Autodesk Fusion 360 part; units mm, degrees
sketch "Sketch2" plane through (0, 0, 0) normal (0, 0, -1) x (1, 0, 0)
  arc A0 (124, -92) -> (125, -91) centre (124, -91) ccw
  line L0 (125, -91) -> (125, -1)
  arc A1 (125, -1) -> (124, 0) centre (124, -1) ccw
  line L1 (124, 0) -> (1, 0)
  arc A2 (1, 0) -> (0, -1) centre (1, -1) ccw
  line L2 (0, -1) -> (0, -91)
  arc A3 (0, -91) -> (1, -92) centre (1, -91) ccw
  line L3 (1, -92) -> (124, -92)
  circle A4 centre (54.1, -72.1) radius 1
  circle A5 centre (11, -21.3) radius 1
  circle A6 centre (26.2, -72.1) radius 1
  circle A7 centre (59.2, -20) radius 1
extrude "Extrude1" add sketch "Sketch2" along normal blind 6
sketch "Sketch1" plane through (0, 0, -6) normal (0, 0, -1) x (1, 0, 0)
  circle A0 centre (59.2, -20) radius 1
  circle A1 centre (11, -21.3) radius 1
  circle A2 centre (26.2, -72.1) radius 1
  circle A3 centre (54.1, -72.1) radius 1
  line L0 (1, -92) -> (124, -92)
  arc A4 (124, -92) -> (125, -91) centre (124, -91) ccw
  line L1 (125, -91) -> (125, -1)
  arc A5 (125, -1) -> (124, 0) centre (124, -1) ccw
  line L2 (124, 0) -> (1, 0)
  arc A6 (1, 0) -> (0, -1) centre (1, -1) ccw
  line L3 (0, -1) -> (0, -91)
  arc A7 (0, -91) -> (1, -92) centre (1, -91) ccw
  line L4 (0, -15) -> (125, -15)
  line L5 (125, -15) -> (125, -25)
  line L6 (125, -25) -> (0, -25)
  line L7 (0, -25) -> (0, -15)
  line L8 (0, -67) -> (125, -67)
  line L9 (125, -67) -> (125, -77)
  line L10 (125, -77) -> (0, -77)
  line L11 (0, -77) -> (0, -67)
  dimension "d215" = 15
  dimension "d216" = 10
  dimension "d217" = 15
  dimension "d218" = 10
extrude "Extrude2" cut sketch "Sketch1" against normal blind 3 contours L1 L3 L8 L9 L10 L11 | L1 L3 L4 L5 L6 L7
fillet "Fillet1" radius 3 1 edges at (125, 20, -3)
fillet "Fillet2" radius 3 1 edges at (125, 72, -3)
fillet "Fillet3" radius 3 1 edges at (0, 72, -3)
fillet "Fillet4" radius 3 1 edges at (0, 20, -3)
delete_face "DeleteFace1" 1 faces at (60.1215, 19.6116, -2)
delete_face "DeleteFace2" 1 faces at (11.995, 21.3996, -1)
delete_face "DeleteFace3" 1 faces at (25.2198, 71.9019, -2)
delete_face "DeleteFace4" 1 faces at (55.0691, 71.8532, -2)
hole "Hole1" at (62.5, 46, 0) direction (0, 0, -1) diameter 2.5 end through all countersink diameter 7.5 countersink angle 90
hole "Hole2" at (62.5, 7.5, 0) direction (0, 0, -1) diameter 2.5 end through all countersink diameter 7.5 countersink angle 90
hole "Hole3" at (62.5, 84.5, 0) direction (0, 0, -1) diameter 2.5 end through all countersink diameter 7.5 countersink angle 90
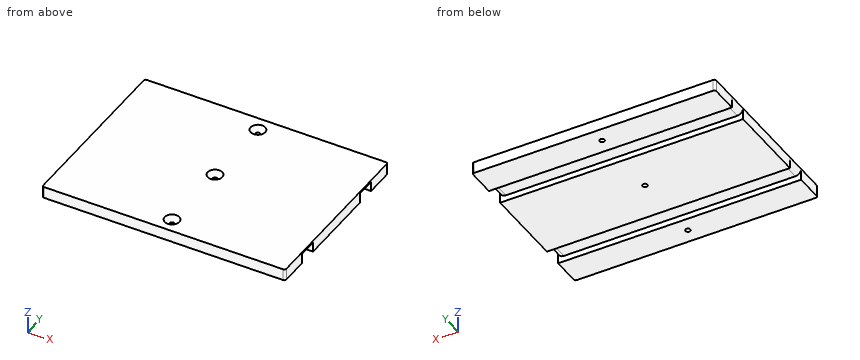
Geometry: final body of the model. Coordinates: model frame, mm. Round coordinates to 2 decimals unless told otherwise and drop trailing zeros. Order: outer loops, then holes, each group sorted by start corner. A loop starts at its lowest first (then second) coordinate and runs counter-clockwise, first axis right, second up. Notation, with made-up numbers: M -21.5,75.5 L 6.5,75.5 A14 cw 6.5,100.5 Z; hole C 5.5,-22 d10. An arc over 180 degrees is marked long. One line per item, written item: value.
(1) Cut plane B-B (y = 46). Return the cut outline in (x, z), and give its area (3 significant figures).
Result sheet:
outline: M 0,-6 L 61.25,-6 L 61.25,-2.5 L 58.75,0 L 0,0 Z; M 63.75,-6 L 125,-6 L 125,0 L 66.25,0 L 63.75,-2.5 Z
area: 729 mm2
(2) Pin query (flat end, axial travel): P1, Ø2, axis at x = 62.5, y = 46, coming from the -Z side; P2, Ø8, axis at x = 60.5, y = 72.5, coming from the -Z side; P3, Ø4, axis at x = 62.5, y = 84.5, coming from the +Z side. Return the tip coordinate at first contact, or that it passes through.
Result sheet:
P1: through
P2: z = -3
P3: z = -1.75
(3) Cut plane D-D (x = 49.5). Return the cut outline in (y, z).
Result sheet:
outline: M 0,-6 L 15,-6 L 15,-3 L 25,-3 L 25,-6 L 67,-6 L 67,-3 L 77,-3 L 77,-6 L 92,-6 L 92,0 L 0,0 Z
(4) Cut plane A-A (z = -3.95). Return the cut outline in (x, y), and give its area (3 significant figures).
Result sheet:
outline: M 0,1 A1 ccw 1,0 L 124,0 A1 ccw 125,1 L 125,15 L 0,15 Z; M 0,25 L 125,25 L 125,67 L 0,67 Z; M 0,77 L 125,77 L 125,91 A1 ccw 124,92 L 1,92 A1 ccw 0,91 Z; hole C 62.5,7.5 d2.5; hole C 62.5,46 d2.5; hole C 62.5,84.5 d2.5
area: 8,980 mm2
(5) Cut plane C-C (x = 62.5). Give the number of separate pieces and of enclosed holes in the cut face, and give its area (3 significant figures).
Result sheet:
separate pieces: 4
enclosed holes: 0
area: 428 mm2
(6) Line query: probe 1 along Y at (x, z) = (62.5, -4.95); probe 2 along Y at (x, z) = (39.5, -3.1); probe 3 along X at (y, z) = (46, -3.25). Output: solid intervals per line, ascending. Write a range as [from, to].
Result sheet:
probe 1: [0, 6.25], [8.75, 15], [25, 44.75], [47.25, 67], [77, 83.25], [85.75, 92]
probe 2: [0, 15], [25, 67], [77, 92]
probe 3: [0, 61.25], [63.75, 125]
